Design review of the part built by this model. Coordinates are the model's own, in mm. Face numbers are marked on the shaded views. Give positions to 0.01 mm unless a question says otherwise; leave off trailing zeros. Order: outer loops, then holes, each group sorted by start corner. A loop starts at its lowest first (then second) coordinate and runs counter-clockwise, first axis right, second up. Notation, with made-up numbers: (22.25, 24.5) -> (70.25, 24.5) arc R22 cw to (70.25, 48.5) -> close; hole circle Ø3 at (-11.75, 30). An arc over 180 degrees is marked (long way). Answer in a Markdown table with one row per item. Add a question column.
```python
from build123d import *

# Parameters (mm, degrees)
SKETCH1_R           = 16.764
BOSS_EXTRUDE1_DEPTH = 57.531
SKETCH3_R           = 21.59
BOSS_EXTRUDE2_DEPTH = 7.62
SKETCH5_R           = 20.32
SKETCH6_R           = 20.32
BOSS_EXTRUDE3_DEPTH = 7.62
CIRPATTERN1_COUNT   = 2
SKETCH9_R           = 16.764
BOSS_EXTRUDE4_DEPTH = 127


with BuildPart() as part:
    # Sketch1 → Boss-Extrude1 (new, symmetric)
    with BuildSketch(Plane(origin=(0, 0, 0), x_dir=(1, 0, 0), z_dir=(0, 1, 0))):
        with Locations(Location((0, 0, 0), (0, 0, 90))):
            Circle(SKETCH1_R)
    extrude(amount=BOSS_EXTRUDE1_DEPTH, both=True)

    # Sketch3 → Boss-Extrude2 (add)
    with BuildSketch(Plane(origin=(0, 57.531, 0), x_dir=(1, 0, 0), z_dir=(0, 1, 0))):
        with Locations(Location((0, 0, 0), (0, 0, 90))):
            Circle(SKETCH3_R)
    boss_extrude2 = extrude(amount=BOSS_EXTRUDE2_DEPTH)

    # Sweep1: sweep along a path in Sketch4
    with BuildLine(Plane.XY) as sweep1_path:
        ThreePointArc((0, 65.151), (8.927385309, 86.703614691), (30.48, 95.631))
    # Sketch5 → Sweep1 (sweep)
    with BuildSketch(Plane(origin=(0, 65.151, 0), x_dir=(1, 0, 0), z_dir=(0, 1, 0))):
        Circle(SKETCH5_R)
    sweep1 = sweep(path=sweep1_path.line)

    # Sketch6 → Boss-Extrude3 (add)
    with BuildSketch(Plane(origin=(30.48, 0, 0), x_dir=(0, 0, -1), z_dir=(1, 0, 0))):
        with Locations(Location((0, 95.631, 0), (0, 0, 90))):
            Circle(SKETCH6_R)
    boss_extrude3 = extrude(amount=BOSS_EXTRUDE3_DEPTH)

    # CirPattern1: Boss-Extrude2, Sweep1, Boss-Extrude3 ×2 about axis
    cirpattern1_axis = Axis((0, 0, 0), (0, 0, 1))
    add([boss_extrude2.rotate(cirpattern1_axis, i * 360 / CIRPATTERN1_COUNT) for i in range(1, CIRPATTERN1_COUNT)])
    add([sweep1.rotate(cirpattern1_axis, i * 360 / CIRPATTERN1_COUNT) for i in range(1, CIRPATTERN1_COUNT)])
    add([boss_extrude3.rotate(cirpattern1_axis, i * 360 / CIRPATTERN1_COUNT) for i in range(1, CIRPATTERN1_COUNT)])

    # Sketch9 → Boss-Extrude4 (add)
    with BuildSketch(Plane(origin=(38.1, 0, 0), x_dir=(0, 0, -1), z_dir=(1, 0, 0))):
        with Locations(Location((0, 95.631, 0), (0, 0, 90))):
            Circle(SKETCH9_R)
    extrude(amount=BOSS_EXTRUDE4_DEPTH)


solid = part.part
```
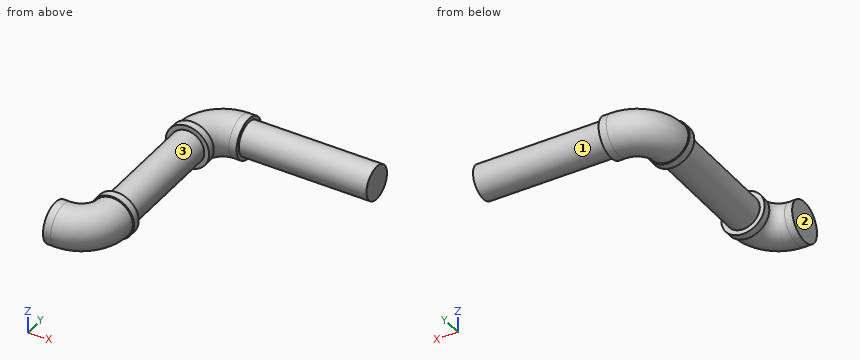
1) Add section B-B, the plane x = 60. Write out the cut boundary in (y, z) (3 decimals).
2) Add section C-C, the plane y = -32. Write out the cut boundary in (x, z).
3) Add section D-D, the plane z = 14. Write out the cut boundary in (x, y).
4) For L1, parallel to Y at x = 5.5, z = 16; L2, parallel to X at y = 96.5, z = -9.5; L3, parallel to Y at x = 93.5, z = -5, list the stretches that pass through material, from the lowest coordinate up.
5) Mouldability with a two-part tool opening along Y and no side actions: class the marked faces 1, 2 and 3 as +Y half, -Y half, draft (parallel to the pull), parting line (faces both ways), or undercut.
6) Add section A-A, the plane z = 0. Write out the cut boundary in (x, y) (3 decimals), and give its area (3 significant figures).
7) Clearance check with flat-ended pins moving along their axes: P1, Ø1.5, axis at y = -52, z = -14.5, coming from the +X side; P2, Ø10, axis at x = 84, z = -7, coming from the +Y side; P3, Ø3, axis at x = 114, z = -9.5, coming from the +Y side. State where each tip first meets the part, or that it passes through.
Verdict:
| question | item | result |
|---|---|---|
| 1 | outline | circle Ø33.528 at (95.631, 0) |
| 2 | outline | circle Ø33.53 at (0, 0) |
| 3 | outline | (-38.1, -110.36) -> (-30.48, -110.36) arc R45.21 ccw to (14.73, -65.15) -> (16.44, -65.15) -> (16.44, -57.53) -> (9.22, -57.53) -> (9.22, 57.53) -> (16.44, 57.53) -> (16.44, 65.15) -> (14.73, 65.15) arc R15.75 cw to (30.48, 80.9) -> (38.1, 80.9) -> (38.1, 86.41) -> (165.1, 86.41) -> (165.1, 104.85) -> (38.1, 104.85) -> (38.1, 110.36) -> (30.48, 110.36) arc R45.21 ccw to (-14.73, 65.15) -> (-16.44, 65.15) -> (-16.44, 57.53) -> (-9.22, 57.53) -> (-9.22, -57.53) -> (-16.44, -57.53) -> (-16.44, -65.15) -> (-14.73, -65.15) arc R15.75 cw to (-30.48, -80.9) -> (-38.1, -80.9) -> close |
| 4 | L1 | y = -88.71 to -57.53, 57.53 to 100.16 |
| 4 | L2 | x = -6.45 to 165.1 |
| 4 | L3 | y = 79.63 to 111.63 |
| 5 | face 1 | parting line |
| 5 | face 2 | draft |
| 5 | face 3 | undercut |
| 6 | outline | (-38.1, -115.951) -> (-30.48, -115.951) arc R50.8 ccw to (20.32, -65.151) -> (21.59, -65.151) -> (21.59, -57.531) -> (16.764, -57.531) -> (16.764, 57.531) -> (21.59, 57.531) -> (21.59, 65.151) -> (20.32, 65.151) arc R10.16 cw to (30.48, 75.311) -> (38.1, 75.311) -> (38.1, 78.867) -> (165.1, 78.867) -> (165.1, 112.395) -> (38.1, 112.395) -> (38.1, 115.951) -> (30.48, 115.951) arc R50.8 ccw to (-20.32, 65.151) -> (-21.59, 65.151) -> (-21.59, 57.531) -> (-16.764, 57.531) -> (-16.764, -57.531) -> (-21.59, -57.531) -> (-21.59, -65.151) -> (-20.32, -65.151) arc R10.16 cw to (-30.48, -75.311) -> (-38.1, -75.311) -> close |
| 6 | area | 13,300 mm2 |
| 7 | P1 | stops at x = 9.59 |
| 7 | P2 | stops at y = 112.28 |
| 7 | P3 | stops at y = 110.36 |
